Here's how the part is built. I have some questions about the finished solid (model axes, mm). Coordinates: 2 decimals unless noted, no trailing zeros. Write each loop counter-clockwise with the first axis right and the second up, starting at its lowest first coordinate (ties: lowest second). Pieces come first, ordered by that corner, then holes.
Item 1: I'm going to push flat-ended pins straight in: pin 1 Ø1.5 at (x, z) = (10.5, 0.5) entering from +Y; pin 2 Ø1 at (x, z) = (15, -1) entering from -Y. Where does each tip first touch, or does it pass through?
Item 2: If I drill on line 1 (Z direction, x = 13, y = -1.25); line 2 (Z direction, x = 15.25, y = 0.5), over which ranges is the centre line in solid material (lowest first)?
Item 3: If we section it at B-B (x = 13): Please give me the cut outline in (y, z) (1 decimal), then the cut area to 3 significant figures.
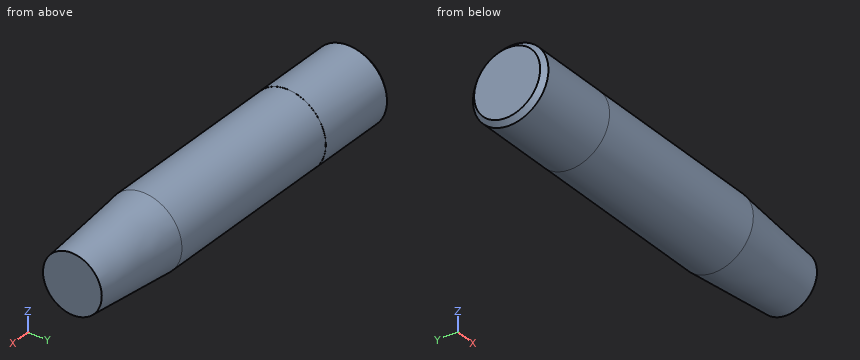
from build123d import *

# Parameters (mm, degrees)
FILLET1_R = 0.25


with BuildPart() as part:
    # Sketch1 → Revolve1 (revolve)
    with BuildSketch(Plane.XY, mode=Mode.PRIVATE) as revolve1_sk:
        Polygon((0, 2.0025), (0, 3.5), (-1, 3.5), (-1, 0), (19.5, 0), (19.5, 1.560056682), (14.5, 1.9975), (4.5, 1.9975), (4.5, 2.0025), align=None)
    revolve(revolve1_sk.sketch.rotate(Axis((-30.167084044, 0, 0), (1, 0, 0)), 90), axis=Axis((-30.167084044, 0, 0), (1, 0, 0)))  # turned: the seam where the file's is

    # Fillet1
    fillet1_edges = [part.edges().sort_by_distance(p)[0] for p in [
        (0, 0, -2.0025),
    ]]
    fillet(fillet1_edges, radius=FILLET1_R)

    # Sketch2 → Cut-Revolve1 (revolve, cut)
    with BuildSketch(Plane.XY, mode=Mode.PRIVATE) as cut_revolve1_sk:
        Polygon((0.25, 2.0025), (0, 1.7525), (0, 0), (-1, 0), (-1, 3.5), (0, 3.5), align=None)
    revolve(cut_revolve1_sk.sketch.rotate(Axis((0, 0, 0), (-1, 0, 0)), 270), axis=Axis((0, 0, 0), (-1, 0, 0)), mode=Mode.SUBTRACT)  # turned: the seam where the file's is


solid = part.part
Answer list:
1. pin 1: stops at y = 2
1. pin 2: stops at y = -1.9
2. line 1: z = -1.56 to 1.56
2. line 2: z = -1.87 to 1.87
3. outline: circle Ø4 at (0, 0)
3. area: 12.5 mm2
